from build123d import *

# Parameters (mm, degrees)
SKETCH_1_W          = 15
SKETCH_1_H          = 15
SKETCH_1_W_2        = 13
SKETCH_1_H_2        = 13
EXTRUDE_1_DEPTH     = 280
SKETCH_2_R          = 1.5
CUT_EXTRUDE_1_DEPTH = 281.501782526
SKETCH_3_R          = 1.5
CUT_EXTRUDE_2_DEPTH = 281.501782526


with BuildPart() as part:
    # 草图1 → 凸台-拉伸1 (new body)
    with BuildSketch(Plane(origin=(0, 0, 0), x_dir=(1, 0, 0), z_dir=(0, 1, 0))):
        Rectangle(SKETCH_1_W, SKETCH_1_H)
        Rectangle(SKETCH_1_W_2, SKETCH_1_H_2, mode=Mode.SUBTRACT)
    extrude(amount=EXTRUDE_1_DEPTH)

    # 草图2 → 切除-拉伸1 (cut, through all)
    with BuildSketch(Plane.XY.offset(7.5)):
        with Locations((0, 40)):
            Circle(SKETCH_2_R)
        with Locations((0, 140)):
            Circle(SKETCH_2_R)
        with Locations((0, 90)):
            Circle(SKETCH_2_R)
        with Locations((0, 240)):
            Circle(SKETCH_2_R)
        with Locations((0, 190)):
            Circle(SKETCH_2_R)
    extrude(amount=-CUT_EXTRUDE_1_DEPTH, mode=Mode.SUBTRACT)

    # 草图3 → 切除-拉伸2 (cut, through all)
    with BuildSketch(Plane(origin=(7.5, 0, 0), x_dir=(0, 0, -1), z_dir=(1, 0, 0))):
        with Locations((0, 160)):
            Circle(SKETCH_3_R)
        with Locations(Location((0, 120, 0), (0, 0, 180))):
            Circle(SKETCH_3_R)
        with Locations((0, 15)):
            Circle(SKETCH_3_R)
        with Locations(Location((0, 265, 0), (0, 0, 180))):
            Circle(SKETCH_3_R)
    extrude(amount=-CUT_EXTRUDE_2_DEPTH, mode=Mode.SUBTRACT)


solid = part.part
Could you check a few things on this model? Use its own coordinates, in mm. A direction names the side the tool comes from. Give positions to 0.01 mm unless a question says otherwise; leave off trailing zeros. Order: outer loops, then holes, each group sorted by start corner. A loop starts at its lowest first (then second) coordinate and runs counter-clockwise, first axis right, second up. Notation, with made-up numbers: (9, 18) - (17, 18) arc R21 ccw to (17, 28) - close; hole circle Ø4 at (-24, 89). An arc over 180 degrees is marked (long way). One line per item, written item: value. Start each with the question number.
1. For P1, Ø2.5, axis at y = 120, z = 0, coming from the +X side; P2, Ø4, axis at y = 265, z = 0, coming from the -X side, each with a flat end and sliding along its axis, tell me the tip position at first contact or that it passes through.
2. If I drill on probe 1 along Y at (x, z) = (0, -6.8); probe 2 along X at (y, z) = (262, -1), over which ranges is the centre line in solid material (lowest first)?
3. Thinking about a two-plate mould opening in X: for faces 1 (the face through (-7.5, 138, 0)), 2 (the face through (-7, 0, 0)), 3 (the face through (7.5, 138, 0)), 4 (the face through (0, 138, -6.5)), which applies, +X half, -X half, draft (parallel to the pull), parting line (faces both ways), or undercut?
4. Imagine slicing it at A-A on z = -4. List the corners of the cut face in (x, y) for me, plus the area to 3 significant figures.
5. Imagine slicing it at B-B on y = 71. List the corners of the cut face in (x, z) for me, plus the area to 3 significant figures.
6. For faces 5 (the face through (0, 138, -7.5)), 6 (the face through (-6.5, 138, 0)), which set-ups out of +Z, -Z, +X, -X, +Y, -Y let a thin tool reach every point of the face, with its end or its side?
Values:
1. P1: through
1. P2: x = -7.5
2. probe 1: 0 to 38.5, 41.5 to 88.5, 91.5 to 138.5, 141.5 to 188.5, 191.5 to 238.5, 241.5 to 280
2. probe 2: -7.5 to -6.5, 6.5 to 7.5
3. face 1: -X half
3. face 2: draft
3. face 3: +X half
3. face 4: undercut
4. outline: (-7.5, 0) - (-6.5, 0) - (-6.5, 280) - (-7.5, 280) - close; (6.5, 0) - (7.5, 0) - (7.5, 280) - (6.5, 280) - close
4. area: 560 mm²
5. outline: (-7.5, -7.5) - (7.5, -7.5) - (7.5, 7.5) - (-7.5, 7.5) - close; hole (-6.5, -6.5) - (6.5, -6.5) - (6.5, 6.5) - (-6.5, 6.5) - close
5. area: 56.0 mm²
6. face 5: -Z, +X, -X, +Y, -Y
6. face 6: +Y, -Y
